Could you check a few things on this model? Use its own coordinates, in mm. A direction names the side the tool comes from. Coordinates: 2 decimals unless noted, no trailing zeros. Write each loop counter-clockwise with the first axis right and the second up, starting at its lowest first coordinate (ties: lowest second). Pieces come first, ordered by that corner, then holes.
```python
from build123d import *

# Parameters (mm, degrees)
SKETCH4_W               = 10
SKETCH4_H               = 13
CUT_EXTRUDE2_DEPTH      = 1
M6_TAPPED_HOLE1_D       = 5
M6_TAPPED_HOLE1_DEPTH   = 10
M6_TAPPED_HOLE1_TIP     = 1.502151548
SKETCH8_R               = 1
CUT_EXTRUDE3_DEPTH      = 7.5
CUT_EXTRUDE3_DEPTH_BACK = 7.5
CHAMFER1_SIZE           = 0.5


with BuildPart() as part:
    # Sketch1 → Revolve1 (revolve)
    with BuildSketch(Plane.XY):
        Polygon((-97, 0), (-97, 4), (-92, 4), (-92, 5), (-3.5, 5), (-3.5, 6), (-2, 6), (-2, 6.5), (0, 6.5), (0, 0), align=None)
    revolve(axis=Axis((0, 0, 0), (1, 0, 0)))

    # Sketch4 → Cut-Extrude2 (cut)
    with BuildSketch(Plane(origin=(0, 0, 0), x_dir=(0, 0, -1), z_dir=(1, 0, 0))):
        Rectangle(SKETCH4_W, SKETCH4_H)
    extrude(amount=-CUT_EXTRUDE2_DEPTH, mode=Mode.SUBTRACT)

    # M6 Tapped Hole1
    with Locations(Plane(origin=(-1, 0, 0), x_dir=(0, 0, -1), z_dir=(1, 0, 0))):
        with Locations((0, 0)):
            Hole(M6_TAPPED_HOLE1_D / 2, depth=M6_TAPPED_HOLE1_DEPTH)
            with Locations((0, 0, -(M6_TAPPED_HOLE1_DEPTH + M6_TAPPED_HOLE1_TIP / 2))):  # 118° drill point
                Cone(0, M6_TAPPED_HOLE1_D / 2, M6_TAPPED_HOLE1_TIP, mode=Mode.SUBTRACT)

    # Sketch8 → Cut-Extrude3 (cut, two sides)
    with BuildSketch(Plane.XY) as cut_extrude3_sk:
        with Locations((-94.5, 0)):
            Circle(SKETCH8_R)
    extrude(amount=CUT_EXTRUDE3_DEPTH, mode=Mode.SUBTRACT)
    extrude(cut_extrude3_sk.sketch, amount=-CUT_EXTRUDE3_DEPTH_BACK, mode=Mode.SUBTRACT)

    # Chamfer1
    chamfer1_edges = [part.edges().sort_by_distance(p)[0] for p in [
        (-97, -4, 0),
    ]]
    chamfer(chamfer1_edges, length=CHAMFER1_SIZE)


solid = part.part
```
Item 1: I want a section at B-B, the plane x = -94.5. List the corners of the cut face in (y, z) for me.
Item 2: If I drill on line 1 along Y through (x, z) = (-94.5, -1.9); line 2 along Y through (x, z) = (-9, -3); line 3 along X through (y, z) = (1, 4.25), over which ranges is the centre line in solid material (lowest first)?
Item 3: I want a section at C-C, the plane x = -57. List the corners of the cut face in (y, z) for me, then the cut area to 3 significant figures.
Item 4: Which directions (+Z, -Z, +X, -X, +Y, -Y) give clear straight access to the entire face, cutting with the end or side of a thin tool? Please do faces 4 (the cylindrical face through (-6.07, -2.44, -0.54)), 5 (the flat face through (0, 0, 6)), 6 (the flat face through (-2, -2, -6)).
Item 5: If we mould it in two halves opening along Z, with no side actions, what happens to faces 1 (the flat face through (-1, 2, -2)), 2 (the cylindrical face through (-1.21, 6.2, 1.95)), 3 (the flat face through (-97, 0, 0))? For each: released by +Z, released by -Z, zero draft, split by the parting line, or undercut.
Item 6: I want a section at A-A, the plane x = -9.5. List the corners of the cut face in (y, z) for me, then the cut area to 3 significant figures.
Item 7: Will these pins go through, and if not, where does the flat tip stop? pin 1 Ø6.5 at (y, z) = (0, 0) entering from +X; pin 2 Ø1.5 at (x, y) = (-30, -5) entering from +Z; pin 3 Ø1.5 at (x, z) = (-30, 2.5) entering from -Y; pin 4 Ø1.2 at (x, y) = (-94.5, 0) entering from +Z.
Taken from the geometry:
1. outline: (-1, -3.87) - (-1, 3.87) arc R4 ccw to start; (1, -3.87) arc R4 ccw to (1, 3.87) - close
2. line 1: y = -3.52 to -1, 1 to 3.52
2. line 2: y = -4 to 4
2. line 3: x = -92 to -1
3. outline: circle Ø10 at (0, 0)
3. area: 78.5 mm2
4. face 4: +X
4. face 5: +Z, -Z, +X, +Y, -Y
4. face 6: -X
5. face 1: undercut
5. face 2: split by the parting line
5. face 3: zero draft
6. outline: circle Ø10 at (0, 0); hole circle Ø5 at (0, 0)
6. area: 58.9 mm2
7. pin 1: stops at x = -1
7. pin 2: stops at z = 2.63
7. pin 3: stops at y = -4.68
7. pin 4: passes through
